Can you work these out from the model? Positions are in its coordinate system, mm. A direction names the side the tool comes from. Give positions to 0.01 mm unless a question says otherwise; leave off trailing zeros. Write each loop counter-clockwise with the first axis right and the second up, starting at its lowest first coordinate (ties: lowest second). Pieces come first, ordered by that corner, then holes.
```python
from build123d import *

# Parameters (mm, degrees)
SKETCH1_R           = 50
SKETCH1_R_2         = 25
SKETCH1_R_3         = 2.9
BOSS_EXTRUDE1_DEPTH = 3.4
SKETCH2_R           = 50
SKETCH2_R_2         = 27.5
BOSS_EXTRUDE2_DEPTH = 3
SKETCH3_R           = 2
CUT_EXTRUDE1_DEPTH  = 6.4
SKETCH4_R           = 2.75
CUT_EXTRUDE2_DEPTH  = 5


with BuildPart() as part:
    # Sketch1 → Boss-Extrude1 (new body)
    with BuildSketch(Plane(origin=(0, 0, 0), x_dir=(1, 0, 0), z_dir=(0, 1, 0))):
        with Locations(Location((0, 0, 0), (0, 0, 270))):
            Circle(SKETCH1_R)
        with Locations(Location((0, 0, 0), (0, 0, 270))):
            Circle(SKETCH1_R_2, mode=Mode.SUBTRACT)
        with Locations(Location((0, 35, 0), (0, 0, 270))):
            Circle(SKETCH1_R_3, mode=Mode.SUBTRACT)
        with Locations(Location((13.393920133, 32.335783638, 0), (0, 0, 270))):
            Circle(SKETCH1_R_3, mode=Mode.SUBTRACT)
        with Locations(Location((24.748737342, 24.748737342, 0), (0, 0, 270))):
            Circle(SKETCH1_R_3, mode=Mode.SUBTRACT)
        with Locations(Location((32.335783638, 13.393920133, 0), (0, 0, 270))):
            Circle(SKETCH1_R_3, mode=Mode.SUBTRACT)
        with Locations(Location((35, 0, 0), (0, 0, 270))):
            Circle(SKETCH1_R_3, mode=Mode.SUBTRACT)
        with Locations(Location((32.335783638, -13.393920133, 0), (0, 0, 270))):
            Circle(SKETCH1_R_3, mode=Mode.SUBTRACT)
        with Locations(Location((24.748737342, -24.748737342, 0), (0, 0, 270))):
            Circle(SKETCH1_R_3, mode=Mode.SUBTRACT)
        with Locations(Location((13.393920133, -32.335783638, 0), (0, 0, 270))):
            Circle(SKETCH1_R_3, mode=Mode.SUBTRACT)
        with Locations(Location((0, -35, 0), (0, 0, 270))):
            Circle(SKETCH1_R_3, mode=Mode.SUBTRACT)
        with Locations(Location((-13.393920133, -32.335783638, 0), (0, 0, 270))):
            Circle(SKETCH1_R_3, mode=Mode.SUBTRACT)
        with Locations(Location((-24.748737342, -24.748737342, 0), (0, 0, 270))):
            Circle(SKETCH1_R_3, mode=Mode.SUBTRACT)
        with Locations(Location((-32.335783638, -13.393920133, 0), (0, 0, 270))):
            Circle(SKETCH1_R_3, mode=Mode.SUBTRACT)
        with Locations(Location((-35, 0, 0), (0, 0, 270))):
            Circle(SKETCH1_R_3, mode=Mode.SUBTRACT)
        with Locations(Location((-32.335783638, 13.393920133, 0), (0, 0, 270))):
            Circle(SKETCH1_R_3, mode=Mode.SUBTRACT)
        with Locations(Location((-24.748737342, 24.748737342, 0), (0, 0, 270))):
            Circle(SKETCH1_R_3, mode=Mode.SUBTRACT)
        with Locations(Location((-13.393920133, 32.335783638, 0), (0, 0, 270))):
            Circle(SKETCH1_R_3, mode=Mode.SUBTRACT)
    extrude(amount=BOSS_EXTRUDE1_DEPTH)

    # Sketch2 → Boss-Extrude2 (add)
    with BuildSketch(Plane(origin=(0, 3.4, 0), x_dir=(1, 0, 0), z_dir=(0, 1, 0))):
        with Locations(Location((0, 0, 0), (0, 0, 270))):
            Circle(SKETCH2_R)
        with Locations(Location((0, 0, 0), (0, 0, 270))):
            Circle(SKETCH2_R_2, mode=Mode.SUBTRACT)
    extrude(amount=BOSS_EXTRUDE2_DEPTH)

    # Sketch3 → Cut-Extrude1 (cut)
    with BuildSketch(Plane.XZ):
        with Locations(Location((-37.416132554, -25.000660486, 0), (0, 0, 270))):
            Circle(SKETCH3_R)
        with Locations(Location((37.416132554, 25.000660486, 0), (0, 0, 270))):
            Circle(SKETCH3_R)
        with Locations(Location((44.135337618, -8.779064491, 0), (0, 0, 270))):
            Circle(SKETCH3_R)
        with Locations(Location((25.000660486, -37.416132554, 0), (0, 0, 270))):
            Circle(SKETCH3_R)
        with Locations(Location((-8.779064491, -44.135337618, 0), (0, 0, 270))):
            Circle(SKETCH3_R)
        with Locations(Location((-44.135337618, 8.779064491, 0), (0, 0, 270))):
            Circle(SKETCH3_R)
        with Locations(Location((-25.000660486, 37.416132554, 0), (0, 0, 270))):
            Circle(SKETCH3_R)
        with Locations(Location((8.779064491, 44.135337618, 0), (0, 0, 270))):
            Circle(SKETCH3_R)
    extrude(amount=-CUT_EXTRUDE1_DEPTH, mode=Mode.SUBTRACT)

    # Sketch4 → Cut-Extrude2 (cut)
    with BuildSketch(Plane(origin=(0, 6.4, 0), x_dir=(1, 0, 0), z_dir=(0, 1, 0))):
        with Locations(Location((-8.779064491, 44.135337618, 0), (0, 0, 270))):
            Circle(SKETCH4_R)
        with Locations(Location((25.000660486, 37.416132554, 0), (0, 0, 270))):
            Circle(SKETCH4_R)
        with Locations(Location((44.135337618, 8.779064491, 0), (0, 0, 270))):
            Circle(SKETCH4_R)
        with Locations(Location((37.416132554, -25.000660486, 0), (0, 0, 270))):
            Circle(SKETCH4_R)
        with Locations(Location((8.779064491, -44.135337618, 0), (0, 0, 270))):
            Circle(SKETCH4_R)
        with Locations(Location((-25.000660486, -37.416132554, 0), (0, 0, 270))):
            Circle(SKETCH4_R)
        with Locations(Location((-44.135337618, -8.779064491, 0), (0, 0, 270))):
            Circle(SKETCH4_R)
        with Locations(Location((-37.416132554, 25.000660486, 0), (0, 0, 270))):
            Circle(SKETCH4_R)
    extrude(amount=-CUT_EXTRUDE2_DEPTH, mode=Mode.SUBTRACT)


solid = part.part
```
1) Please list where these lines run through material, in increasing order: L1, parallel to X at y = 1.25, z = 26.5; L2, parallel to X at y = 5.5, z = 23; L3, parallel to X at y = 2.5, z = -25.5.
Values follow:
L1: x = -42.4 to -27.06, -22.44 to 22.44, 27.06 to 36.09, 38.74 to 42.4
L2: x = -44.4 to -15.07, 15.07 to 35.53, 39.3 to 44.4
L3: x = -43.01 to -40.12, -34.71 to -27.55, -21.95 to 21.95, 27.55 to 43.01
2) Suppose I cut it at D-D on x = 20. Write out the boundary of the cut face in (y, z), plus the area to 3 significant figures.
Values follow:
outline: (0, -45.83) - (6.4, -45.83) - (6.4, -18.87) - (3.4, -18.87) - (3.4, -15) - (0, -15) - close; (0, 15) - (3.4, 15) - (3.4, 18.87) - (6.4, 18.87) - (6.4, 45.83) - (0, 45.83) - close
area: 371 mm2
3) If we mould it in two halves opening along X, with no side actions, what happens to faces 1 (the face through (42.18, 0.69, -8.35)), 2 (the face through (-22, 6.4, 22))? For each: +X half, -X half, draft (parallel to the pull), parting line (faces both ways), or undercut.
Values follow:
face 1: undercut
face 2: draft
4) Suppose I cut it at A-A on x = 0. Write out the boundary of the cut face in (y, z).
Values follow:
outline: (0, -50) - (6.4, -50) - (6.4, -27.5) - (3.4, -27.5) - (3.4, -25) - (0, -25) - (0, -32.1) - (3.4, -32.1) - (3.4, -37.9) - (0, -37.9) - close; (0, 25) - (3.4, 25) - (3.4, 27.5) - (6.4, 27.5) - (6.4, 50) - (0, 50) - (0, 37.9) - (3.4, 37.9) - (3.4, 32.1) - (0, 32.1) - close
5) For faces 3 (the face through (-40.1, 3.9, -25.6)), 4 (the face through (-31.46, 1.68, -10.63)), 5 (the face through (-39.19, 0.69, -25.924)), which set-ups out of +Z, -Z, +X, -X, +Y, -Y let a thin tool reach every point of the face, with its end or its side?
Values follow:
face 3: +Y
face 4: -Y
face 5: +Y, -Y
6) For pin 1 Ø3 at (x, z) = (13.5, 31) entering from -Y; pin 2 Ø3 at (x, z) = (37.42, 25) entering from -Y; pin 3 Ø3 at (x, y) = (16, 4) entering from +Z, each with a flat end and sliding along its axis, tell me the tip position at first contact or that it passes through.
Values follow:
pin 1: stops at y = 3.4
pin 2: passes through
pin 3: stops at z = 47.85
7) Suppose I cut it at C-C on y = 5.25. State how many separate pieces and enclosed holes the cut face has, plus the area to 3 significant figures.
Values follow:
separate pieces: 1
enclosed holes: 9
area: 5,290 mm2
8) Suppose I cut it at B-B on z = 0. Write out the boundary of the cut face in (x, y), plus the area to 3 significant figures.
Values follow:
outline: (-50, 0) - (-37.9, 0) - (-37.9, 3.4) - (-32.1, 3.4) - (-32.1, 0) - (-25, 0) - (-25, 3.4) - (-27.5, 3.4) - (-27.5, 6.4) - (-50, 6.4) - close; (25, 0) - (32.1, 0) - (32.1, 3.4) - (37.9, 3.4) - (37.9, 0) - (50, 0) - (50, 6.4) - (27.5, 6.4) - (27.5, 3.4) - (25, 3.4) - close
area: 266 mm2
